```python
from build123d import *

# Parameters (mm, degrees)
SKIZZE1_W                       = 62
SKIZZE1_H                       = 48
AUFSATZ_LINEAR_AUSTRAGEN1_DEPTH = 1.5
SKIZZE3_W                       = 4
SKIZZE3_H                       = 4
AUFSATZ_LINEAR_AUSTRAGEN2_DEPTH = 14.8
VERRUNDUNG1_R                   = 1


with BuildPart() as part:
    # Skizze1 → Aufsatz-Linear austragen1 (new body)
    with BuildSketch(Plane.XY):
        with Locations((-8.433613499, 5.076642336)):
            Rectangle(SKIZZE1_W, SKIZZE1_H)
    extrude(amount=AUFSATZ_LINEAR_AUSTRAGEN1_DEPTH)

    # Skizze3 → Aufsatz-Linear austragen2 (add)
    with BuildSketch(Plane.XY.offset(1.5)):
        with Locations((-37.433613499, 27.076642336)):
            Rectangle(SKIZZE3_W, SKIZZE3_H)
        with Locations((-37.433613499, -16.923357664)):
            Rectangle(SKIZZE3_W, SKIZZE3_H)
        with Locations((20.566386501, -6.923357664)):
            Rectangle(SKIZZE3_W, SKIZZE3_H)
    extrude(amount=AUFSATZ_LINEAR_AUSTRAGEN2_DEPTH)

    # Verrundung1
    verrundung1_edges = [part.edges().sort_by_distance(p)[0] for p in [
        (-37.433613499, 25.076642336, 1.5),
        (-35.433613499, 27.076642336, 1.5),
        (-35.433613499, -16.923357664, 1.5),
        (-37.433613499, -14.923357664, 1.5),
        (20.566386501, -4.923357664, 1.5),
        (18.566386501, -6.923357664, 1.5),
        (20.566386501, -8.923357664, 1.5),
    ]]
    fillet(verrundung1_edges, radius=VERRUNDUNG1_R)


solid = part.part
```
Can you work these out from the model? Positions are in its coordinate system, mm. A direction names the side the tool comes from. Round coordinates to 2 decimals unless told otherwise and drop trailing zeros. Loops run counter-clockwise (first coordinate to the right, second up) from the corner with the lowest first, then second, coordinate; pieces in that order, holes last. Notation, with made-up numbers: (45.5, 13) -> (52.5, 13) arc R19 ccw to (52.5, 22) -> close; hole circle Ø5 at (25, 29). An arc over 180 degrees is marked (long way). One line per item, written item: value. Start each with the question number.
1. If we section it at D-D, the plane y = 6.5: Write out the boundary of the cut face in (x, z), then the cut area to 3 significant figures.
2. For pin 1 (6 mm diameter, centred on x = 12, z = 2.5, fed in from -Y); pin 2 (8 mm diameter, centred on y = -9.5, z = 14, fed in from -X); pin 3 (1 mm diameter, centred on x = 6, y = -6.5, fed in from +Z); pin 4 (2 mm diameter, centred on y = 27, z = 10.5, fed in from +X), each with a flat end and sliding along its axis, tell me the tip position at first contact or that it passes through.
3. If we section it at C-C, the plane x = -24: Write out the boundary of the cut face in (y, z), then the cut area to 3 significant figures.
4. For faces 5 (the flat face through (-35.434, 27, 9)), 6 (the flat face through (18.566, -7, 9)), 7 (the flat face through (21, -4.923, 9)), 8 (the flat face through (21, -8.923, 9)), which set-ups out of +Z, -Z, +X, -X, +Y, -Y let a thin tool reach every point of the face, with its end or its side?
5. If we section it at A-A, the plane y = -7.5: Write out the boundary of the cut face in (x, z).
6. If we section it at B-B, the plane z = 10: Write out the boundary of the cut face in (x, y).
7. If I drill on probe 1 along Z at (x, y) = (18, -15.5); probe 2 along Y at (x, z) = (19, 11); probe 3 along X at (y, z) = (-16, 10), over which ranges is the centre line in solid material (lowest first)?
8. If we mould it in two halves opening along Y, with no side actions, what happens to faces 1 (the flat face through (-37, 25.077, 9)), 2 (the flat face through (-20, 29.077, 1)), 3 (the flat face through (-37, -14.923, 9)), 4 (the flat face through (-35.434, -17, 9))? For each: pulls with the +Y half, pulls with the -Y half, needs draft (parallel to the pull), parting line crosses it, or undercut.
Calculated:
1. outline: (-39.43, 0) -> (22.57, 0) -> (22.57, 1.5) -> (-39.43, 1.5) -> close
1. area: 93.0 mm²
2. pin 1: stops at y = -18.92
2. pin 2: stops at x = 18.57
2. pin 3: stops at z = 1.5
2. pin 4: stops at x = -35.43
3. outline: (-18.92, 0) -> (29.08, 0) -> (29.08, 1.5) -> (-18.92, 1.5) -> close
3. area: 72.0 mm²
4. face 5: +Z, +X, +Y, -Y
4. face 6: +Z, -X, +Y, -Y
4. face 7: +Z, +X, -X, +Y
4. face 8: +Z, +X, -X, -Y
5. outline: (-39.43, 0) -> (22.57, 0) -> (22.57, 16.3) -> (18.57, 16.3) -> (18.57, 2.5) arc R1 cw to (17.57, 1.5) -> (-39.43, 1.5) -> close
6. outline: (-39.43, -18.92) -> (-35.43, -18.92) -> (-35.43, -14.92) -> (-39.43, -14.92) -> close; (-39.43, 25.08) -> (-35.43, 25.08) -> (-35.43, 29.08) -> (-39.43, 29.08) -> close; (18.57, -8.92) -> (22.57, -8.92) -> (22.57, -4.92) -> (18.57, -4.92) -> close
7. probe 1: z = 0 to 1.5
7. probe 2: y = -8.92 to -4.92
7. probe 3: x = -39.43 to -35.43
8. face 1: undercut
8. face 2: pulls with the +Y half
8. face 3: undercut
8. face 4: needs draft
